The model under review builds one solid part; all positions refer to its coordinate system, in mm. A direction names the side the tool comes from. Coordinates: 2 decimals unless noted, no trailing zeros. Write each loop counter-clockwise with the first axis right and the second up, starting at its lowest first coordinate (ties: lowest second). Pieces come first, ordered by that corner, then holes. Notation, with made-up numbers: (15.25, -7.5) - (27.25, -7.5) arc R21 cw to (27.25, 5.5) - close; hole circle Ø11 at (-27.75, 36.25). An arc over 180 degrees is marked (long way). Use one line per item in the form item = value. Start each with the question number.
Autodesk Inventor part; units mm, degrees
ref_plane "YZ Plane" through (0, 0, 0) normal (1, 0, 0) x (0, 1, 0)
ref_plane "XZ Plane" through (0, 0, 0) normal (0, 1, 0) x (-1, 0, 0)
ref_plane "XY Plane" through (0, 0, 0) normal (0, 0, 1) x (1, 0, 0)
sketch "スケッチ1" plane through (0, 0, 0) normal (0, 0, 1) x (1, 0, 0)
  circle A0 centre (250, -200) radius 1.6 construction
  circle A1 centre (239, -189) radius 1.6 construction
  circle A2 centre (250, -200) radius 3.2
  circle A3 centre (239, -189) radius 3.2
  circle A4 centre (250, -200) radius 5 construction
  circle A5 centre (239, -189) radius 5 construction
  line L0 (242.5355, -185.4645) -> (253.5355, -196.4645)
  line L1 (250, -200) -> (239, -189) construction
  line L2 (-250, -205) -> (250, -205)
  line L3 (244, -202) -> (234, -202)
  line L4 (234, -202) -> (234, -189)
  line L5 (244, -202) -> (244, -205)
  line L6 (244, -205) -> (250, -205)
  arc A6 (250, -205) -> (253.5355, -196.4645) centre (250, -200) ccw
  arc A7 (242.5355, -185.4645) -> (234, -189) centre (239, -189) ccw
  point P0 (0, 0)
  point P1 (255, -200)
  dimension "d0" = 6.4
  dimension "d2" = 10
  dimension "d3" = 3
extrude "押し出し1" add sketch "スケッチ1" along normal blind 130
sketch "スケッチ2" plane through (234, -202, 0) normal (0, -1, 0) x (1, 0, 0)
  line L0 (1.8, 130) -> (8.2, 130) construction
  line L1 (1.8, 0) -> (8.2, 0) construction
  line L2 (5, 130) -> (5, 0) construction
  circle A0 centre (5, 125) radius 2.25
  circle A1 centre (5, 5) radius 2.25
  point P0 (-234, 0)
  dimension "d6" = 4.5
  dimension "d7" = 5
  dimension "d8" = 5
extrude "押し出し2" cut sketch "スケッチ2" against normal blind 5
sketch "スケッチ3" plane through (234, -202, 0) normal (0, -1, 0) x (1, 0, 0)
  circle A0 centre (5, 125) radius 2.25 construction
  circle A1 centre (5, 5) radius 2.25 construction
  circle A2 centre (5, 125) radius 1.6
  circle A3 centre (5, 5) radius 1.6
  point P0 (-234, 0)
  dimension "d11" = 3.2
extrude "押し出し3" cut sketch "スケッチ3" against normal blind 13
equation "\"d8\" = d7"
properties part number "radiator_adapter_01"
1. Take a section at D-D (x = 252). State the section outline as (y, z) points.
2. The part is to be moulded in two halves that separate along X. For faces 4 (the cylindrical face through (237.011, -184.413, 64.09)), 5 (the cylindrical face through (253.052, -200.961, 64.09)), 6 (the flat face through (247, -205, 64)), say which applies: released by +X, released by -X, zero draft, split by the parting line, or undercut.
3. Take a section at C-C (z = 61). State the section outline as (x, y) points.
4. Take a section at B-B (z = 125). State the section outline as (x, y) points.
5. For faces 1 (the flat face through (239, -197, 127)), 2 (the flat face through (239, -202, 64)), 3 (the cylindrical face through (240.477, -186.161, 64.09)), list the 3-axis set-ups (+Z, -Z, +X, -X, +Y, -Y) from which the entire face can be reached by the end or side of a thin tool; tool diameter is ignored.
6. For L1, parallel to Z at x = 239, y = -193.85; L2, parallel to Z at x = 239, y = -199.9; L3, parallel to X at y = -200, z = 77, list the stretches that pass through material, from the lowest coordinate up.
7. For P1, Ø2.5, axis at x = 239, z = 125, coming from the -Y side; P2, Ø5, axis at y = -192.5, z = 66, coming from the +X side; P3, Ø8, axis at x = 249.5, z = 88.5, coming from the +Y side, all flat-tipped, find the tip position at first contact; note any pin that passes through.
8. Take a section at A-A (y = -200). State the section outline as (x, z) points, plus the area to 3 significant figures.
Returned:
q1.outline = (-204.58, 0) - (-202.5, 0) - (-202.5, 130) - (-204.58, 130) - close; (-197.5, 0) - (-194.93, 0) - (-194.93, 130) - (-197.5, 130) - close
q2.face_4 = split by the parting line
q2.face_5 = undercut
q2.face_6 = zero draft
q3.outline = (234, -202) - (244, -202) - (244, -205) - (250, -205) arc R5 ccw to (253.54, -196.46) - (242.54, -185.46) arc R5 ccw to (234, -189) - close; hole circle Ø6.4 at (239, -189); hole circle Ø6.4 at (250, -200)
q4.outline = (234, -202) - (236.75, -202) - (236.75, -197) - (237.4, -197) - (237.4, -191.77) arc R3.2 cw (long way) to (240.6, -191.77) - (240.6, -197) - (241.25, -197) - (241.25, -202) - (244, -202) - (244, -205) - (250, -205) arc R5 ccw to (253.54, -196.46) - (242.54, -185.46) arc R5 ccw to (234, -189) - close; hole circle Ø6.4 at (250, -200)
q5.face_1 = -Y
q5.face_2 = +Z, -Z, -X, -Y
q5.face_3 = +Z, -Z
q6.L1 = 0 to 3.4, 6.6 to 123.4, 126.6 to 130
q6.L2 = 0 to 2.75, 7.25 to 122.75, 127.25 to 130
q6.L3 = 234 to 246.8, 253.2 to 255
q7.P1 = -186.05
q7.P2 = 252.07
q7.P3 = -188.43
q8.outline = (234, 0) - (246.8, 0) - (246.8, 130) - (234, 130) - close; (253.2, 0) - (255, 0) - (255, 130) - (253.2, 130) - close; hole circle Ø4.5 at (239, 5); hole circle Ø4.5 at (239, 125)
q8.area = 1,870 mm²
